Verification items for the finished model (mm, model axes). Round coordinates to 2 decimals unless told otherwise and drop trailing zeros. Write each loop counter-clockwise with the first axis right and the second up, starting at its lowest first coordinate (ties: lowest second). Pieces come first, ordered by that corner, then holes. Notation, with made-up numbers: (-11, -33) - (17, -33) arc R26 cw to (17, -9) - close; hole circle Ø11 at (38, -7). An arc over 180 degrees is marked (long way). Answer as a JSON object with one key per item and string values.
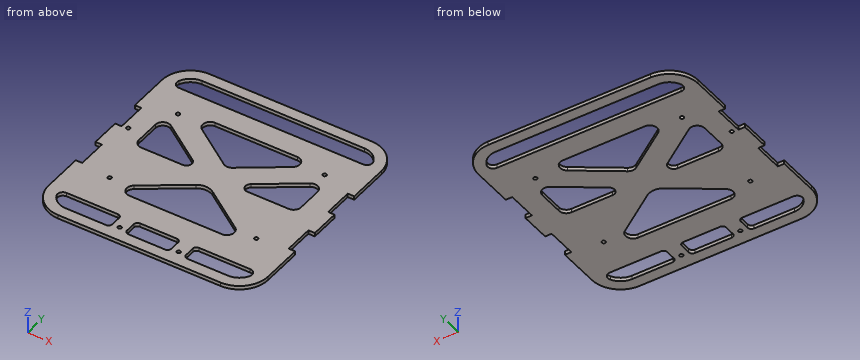
```python
from build123d import *

# Parameters (mm, degrees)
SKETCH1_R           = 1.5875
BOSS_EXTRUDE1_DEPTH = 3.175


with BuildPart() as part:
    # Sketch1 → Boss-Extrude1 (new body)
    with BuildSketch(Plane.XY.offset(-676.275)):
        with BuildLine():
            Line((94.488, -171.45), (94.488, -136.525))
            Line((94.488, -136.525), (88.9, -136.525))
            Line((88.9, -136.525), (88.9, -111.125))
            Line((88.9, -111.125), (94.488, -111.125))
            Line((94.488, -111.125), (94.488, -85.725))
            Line((94.488, -85.725), (88.9, -85.725))
            Line((88.9, -85.725), (88.9, -60.325))
            Line((88.9, -60.325), (94.488, -60.325))
            Line((94.488, -60.325), (94.488, -25.4))
            ThreePointArc((94.488, -25.4), (87.271696875, -7.978303125), (69.85, -0.762))
            Line((69.85, -0.762), (-69.85, -0.762))
            ThreePointArc((-69.85, -0.762), (-87.271696875, -7.978303125), (-94.488, -25.4))
            Line((-94.488, -25.4), (-94.488, -60.325))
            Line((-94.488, -60.325), (-88.9, -60.325))
            Line((-88.9, -60.325), (-88.9, -85.725))
            Line((-88.9, -85.725), (-94.488, -85.725))
            Line((-94.488, -85.725), (-94.488, -111.125))
            Line((-94.488, -111.125), (-88.9, -111.125))
            Line((-88.9, -111.125), (-88.9, -136.525))
            Line((-88.9, -136.525), (-94.488, -136.525))
            Line((-94.488, -136.525), (-94.488, -171.45))
            ThreePointArc((-94.488, -171.45), (-87.271696875, -188.871696875), (-69.85, -196.088))
            Line((-69.85, -196.088), (69.85, -196.088))
            ThreePointArc((69.85, -196.088), (87.271696875, -188.871696875), (94.488, -171.45))
        make_face()
        with Locations(Location((63.1655201, -139.7, 0), (0, 0, 180))):
            Circle(SKETCH1_R, mode=Mode.SUBTRACT)
        with Locations(Location((-83.82, -84.836714101, 0), (0, 0, 180))):
            Circle(SKETCH1_R, mode=Mode.SUBTRACT)
        with Locations(Location((-63.1655201, -51.5992872, 0), (0, 0, 180))):
            Circle(SKETCH1_R, mode=Mode.SUBTRACT)
        with Locations(Location((25.4, -183.388, 0), (0, 0, 180))):
            Circle(SKETCH1_R, mode=Mode.SUBTRACT)
        with Locations(Location((-25.4, -183.388, 0), (0, 0, 180))):
            Circle(SKETCH1_R, mode=Mode.SUBTRACT)
        with Locations(Location((-63.1655201, -139.7, 0), (0, 0, 180))):
            Circle(SKETCH1_R, mode=Mode.SUBTRACT)
        with Locations(Location((63.1655201, -51.5992872, 0), (0, 0, 180))):
            Circle(SKETCH1_R, mode=Mode.SUBTRACT)
        with BuildLine():
            Line((7.264641701, -112.328307791), (43.598023874, -137.666473794))
            ThreePointArc((43.598023874, -137.666473794), (46.023616914, -144.778727737), (39.965703023, -149.225))
            Line((39.965703023, -149.225), (-39.965703023, -149.225))
            ThreePointArc((-39.965703023, -149.225), (-46.023616914, -144.778727737), (-43.598023874, -137.666473794))
            Line((-43.598023874, -137.666473794), (-7.264641701, -112.328307791))
            ThreePointArc((-7.264641701, -112.328307791), (0, -110.045360203), (7.264641701, -112.328307791))
        make_face(mode=Mode.SUBTRACT)
        with BuildLine():
            Line((39.04526783, -56.807813406), (3.632320851, -81.504086518))
            ThreePointArc((3.632320851, -81.504086518), (0, -82.645560312), (-3.632320851, -81.504086518))
            Line((-3.632320851, -81.504086518), (-39.04526783, -56.807813406))
            ThreePointArc((-39.04526783, -56.807813406), (-41.47086087, -49.695559463), (-35.41294698, -45.2492872))
            Line((-35.41294698, -45.2492872), (35.41294698, -45.2492872))
            ThreePointArc((35.41294698, -45.2492872), (41.47086087, -49.695559463), (39.04526783, -56.807813406))
        make_face(mode=Mode.SUBTRACT)
        with BuildLine():
            Line((69.85, -70.72011097), (69.85, -92.075))
            ThreePointArc((69.85, -92.075), (67.990128061, -96.565128061), (63.5, -98.425))
            Line((63.5, -98.425), (27.826758339, -98.425))
            ThreePointArc((27.826758339, -98.425), (23.283322921, -95.090295803), (25.102517701, -89.756105345))
            Line((25.102517701, -89.756105345), (59.867679149, -65.511584764))
            ThreePointArc((59.867679149, -65.511584764), (66.4374532, -65.090380186), (69.85, -70.72011097))
        make_face(mode=Mode.SUBTRACT)
        with BuildLine():
            Line((-59.867679149, -65.511584764), (-25.102517701, -89.756105345))
            ThreePointArc((-25.102517701, -89.756105345), (-23.283322921, -95.090295803), (-27.826758339, -98.425))
            Line((-27.826758339, -98.425), (-63.5, -98.425))
            ThreePointArc((-63.5, -98.425), (-67.990128061, -96.565128061), (-69.85, -92.075))
            Line((-69.85, -92.075), (-69.85, -70.72011097))
            ThreePointArc((-69.85, -70.72011097), (-66.4374532, -65.090380186), (-59.867679149, -65.511584764))
        make_face(mode=Mode.SUBTRACT)
        with BuildLine():
            Line((-69.85, -186.563), (-34.925, -186.563))
            ThreePointArc((-34.925, -186.563), (-32.67993597, -185.63306403), (-31.75, -183.388))
            Line((-31.75, -183.388), (-31.75, -174.625))
            ThreePointArc((-31.75, -174.625), (-32.67993597, -172.37993597), (-34.925, -171.45))
            Line((-34.925, -171.45), (-79.039746678, -171.45))
            ThreePointArc((-79.039746678, -171.45), (-83.108999442, -173.738113573), (-83.268157726, -178.403834356))
            ThreePointArc((-83.268157726, -178.403834356), (-77.702052928, -184.363095439), (-69.85, -186.563))
        make_face(mode=Mode.SUBTRACT)
        with BuildLine():
            Line((69.85, -10.287), (-69.85, -10.287))
            ThreePointArc((-69.85, -10.287), (-78.244855824, -12.833012903), (-83.811231367, -19.613223028))
            ThreePointArc((-83.811231367, -19.613223028), (-83.371868677, -24.08222496), (-79.411683667, -26.1992872))
            Line((-79.411683667, -26.1992872), (79.411683667, -26.1992872))
            ThreePointArc((79.411683667, -26.1992872), (83.371868677, -24.08222496), (83.811231367, -19.613223028))
            ThreePointArc((83.811231367, -19.613223028), (78.244855824, -12.833012903), (69.85, -10.287))
        make_face(mode=Mode.SUBTRACT)
        with BuildLine():
            Line((-19.05, -183.388), (-19.05, -174.625))
            ThreePointArc((-19.05, -174.625), (-18.12006403, -172.37993597), (-15.875, -171.45))
            Line((-15.875, -171.45), (15.875, -171.45))
            ThreePointArc((15.875, -171.45), (18.12006403, -172.37993597), (19.05, -174.625))
            Line((19.05, -174.625), (19.05, -183.388))
            ThreePointArc((19.05, -183.388), (18.12006403, -185.63306403), (15.875, -186.563))
            Line((15.875, -186.563), (-15.875, -186.563))
            ThreePointArc((-15.875, -186.563), (-18.12006403, -185.63306403), (-19.05, -183.388))
        make_face(mode=Mode.SUBTRACT)
        with BuildLine():
            Line((31.75, -174.625), (31.75, -183.388))
            ThreePointArc((31.75, -183.388), (32.67993597, -185.63306403), (34.925, -186.563))
            Line((34.925, -186.563), (69.85, -186.563))
            ThreePointArc((69.85, -186.563), (77.702052928, -184.363095439), (83.268157726, -178.403834356))
            ThreePointArc((83.268157726, -178.403834356), (83.108999442, -173.738113573), (79.039746678, -171.45))
            Line((79.039746678, -171.45), (34.925, -171.45))
            ThreePointArc((34.925, -171.45), (32.67993597, -172.37993597), (31.75, -174.625))
        make_face(mode=Mode.SUBTRACT)
    extrude(amount=-BOSS_EXTRUDE1_DEPTH)


solid = part.part
```
1. Go/stop test with flat-tipped pins: pin 1 (1 mm diameter, centred on y = -77.5, z = -677.5, fed in from +X); pin 2 (1.6 mm diameter, centred on x = -92.5, z = -678, fed in from -Y); pin 3 (1.6 mm diameter, centred on y = -73.5, z = -677.5, fed in from -X); pin 4 (1.9 mm diameter, centred on x = -63.17, y = -139.7, fed in from +Z). Record where each tip stops, or that it passes through.
Completed:
{"pin 1": "stops at x = 88.9", "pin 2": "stops at y = -182.83", "pin 3": "stops at x = -88.9", "pin 4": "passes through"}
2. Cross-section at C-C (z = -677.5). Count the separate pieces of the cut face and the enclosed holes in it, plus the area to 3 significant figures.
Completed:
{"separate pieces": "1", "enclosed holes": "15", "area": "24,700 mm^2"}
3. Material ranges on probe 1 along X at (y, z) = (-173.5, -678.25); probe 2 along Y at (x, z) = (-35.5, -679.15) (3 decimals); probe 3 along X at (y, z) = (-182.5, -676.9), recorded low to high. Write a range as from..to.
Completed:
{"probe 1": "x = -94.4..-82.95, -31.96..-18.84, 18.84..31.96, 82.95..94.4", "probe 2": "y = -196.088..-186.563, -171.45..-149.225, -132.019..-98.425, -82.505..-59.28, -45.25..-26.199, -10.287..-0.762", "probe 3": "x = -91.87..-80.16, -31.75..-26.72, -24.08..-19.05, 19.05..24.08, 26.72..31.75, 80.16..91.87"}
4. Cross-section at B-B (x = -54.5). Record the boundary of the cut face in (y, z) (3 decimals), plus the area to 3 significant figures.
Completed:
{"outline": "(-196.088, -679.45) - (-186.563, -679.45) - (-186.563, -676.275) - (-196.088, -676.275) - close; (-171.45, -679.45) - (-98.425, -679.45) - (-98.425, -676.275) - (-171.45, -676.275) - close; (-69.255, -679.45) - (-26.199, -679.45) - (-26.199, -676.275) - (-69.255, -676.275) - close; (-10.287, -679.45) - (-0.762, -679.45) - (-0.762, -676.275) - (-10.287, -676.275) - close", "area": "429 mm^2"}
5. Cross-section at A-A (x = 74). Record the boundary of the cut face in (y, z) (3 decimals).
Completed:
{"outline": "(-195.736, -679.45) - (-185.982, -679.45) - (-185.982, -676.275) - (-195.736, -676.275) - close; (-171.45, -679.45) - (-26.199, -679.45) - (-26.199, -676.275) - (-171.45, -676.275) - close; (-10.868, -679.45) - (-1.114, -679.45) - (-1.114, -676.275) - (-10.868, -676.275) - close"}
